Verification items for the finished model (mm, model axes). Give positions to 0.01 mm unless a question says otherwise; leave off trailing zeros. Write each loop counter-clockwise with the first axis right and the second up, starting at its lowest first coordinate (ties: lowest second). Pieces come first, ordered by that corner, then holes. Notation, with made-up numbers: M -8,3 L 44,3 A22 ccw 44,21 Z; hole C 17.25,35 d10. An arc over 180 degrees is marked long. Answer as a JSON object with one key per item and string values.
```python
from build123d import *

# Parameters (mm, degrees)
SKETCH1_R           = 2.54
BOSS_EXTRUDE1_DEPTH = 2.286
SKETCH2_W           = 25.4
SKETCH2_H           = 31.75
CUT_EXTRUDE1_DEPTH  = 2.54
FILLET1_R           = 6.35


with BuildPart() as part:
    # Sketch1 → Boss-Extrude1 (new body)
    with BuildSketch(Plane(origin=(0, 0, 0), x_dir=(1, 0, 0), z_dir=(0, 1, 0))):
        Polygon((25.4, 114.3), (0, 114.3), (0, 0), (25.4, 0), (25.4, 31.75), (69.85, 31.75), (69.85, 82.55), (25.4, 82.55), align=None)
        with Locations(Location((12.7, 95.25, 0), (0, 0, 270))):
            Circle(SKETCH1_R, mode=Mode.SUBTRACT)
        with Locations(Location((12.7, 69.85, 0), (0, 0, 270))):
            Circle(SKETCH1_R, mode=Mode.SUBTRACT)
        with Locations(Location((12.7, 44.45, 0), (0, 0, 270))):
            Circle(SKETCH1_R, mode=Mode.SUBTRACT)
        with Locations(Location((12.7, 19.05, 0), (0, 0, 270))):
            Circle(SKETCH1_R, mode=Mode.SUBTRACT)
        with Locations(Location((38.1, 69.85, 0), (0, 0, 270))):
            Circle(SKETCH1_R, mode=Mode.SUBTRACT)
        with Locations(Location((50.8, 69.85, 0), (0, 0, 270))):
            Circle(SKETCH1_R, mode=Mode.SUBTRACT)
        with Locations(Location((63.5, 69.85, 0), (0, 0, 270))):
            Circle(SKETCH1_R, mode=Mode.SUBTRACT)
        with Locations(Location((50.8, 57.15, 0), (0, 0, 270))):
            Circle(SKETCH1_R, mode=Mode.SUBTRACT)
        with Locations(Location((63.5, 57.15, 0), (0, 0, 270))):
            Circle(SKETCH1_R, mode=Mode.SUBTRACT)
        with Locations(Location((50.8, 44.45, 0), (0, 0, 270))):
            Circle(SKETCH1_R, mode=Mode.SUBTRACT)
        with Locations(Location((63.5, 44.45, 0), (0, 0, 270))):
            Circle(SKETCH1_R, mode=Mode.SUBTRACT)
        with Locations(Location((38.1, 57.15, 0), (0, 0, 270))):
            Circle(SKETCH1_R, mode=Mode.SUBTRACT)
        with Locations(Location((38.1, 44.45, 0), (0, 0, 270))):
            Circle(SKETCH1_R, mode=Mode.SUBTRACT)
    extrude(amount=BOSS_EXTRUDE1_DEPTH)

    # Sketch2 → Cut-Extrude1 (cut)
    with BuildSketch(Plane(origin=(0, 2.286, 0), x_dir=(1, 0, 0), z_dir=(0, 1, 0))):
        with Locations((12.7, 98.425)):
            Rectangle(SKETCH2_W, SKETCH2_H)
    extrude(amount=-CUT_EXTRUDE1_DEPTH, mode=Mode.SUBTRACT)

    # Fillet1
    fillet1_edges = [part.edges().sort_by_distance(p)[0] for p in [
        (69.85, 1.143, -82.55),
        (69.85, 1.143, -31.75),
        (25.4, 1.143, -31.75),
        (25.4, 1.143, 0),
        (0, 1.143, 0),
        (0, 1.143, -82.55),
    ]]
    fillet(fillet1_edges, radius=FILLET1_R)


solid = part.part
```
1) Section check B-B on z = -44.45. Record the boundary of the cut face in (x, y), and give its area (3 significant figures).
Completed:
{"outline": "M 0,0 L 10.16,0 L 10.16,2.29 L 0,2.29 Z; M 15.24,0 L 35.56,0 L 35.56,2.29 L 15.24,2.29 Z; M 40.64,0 L 48.26,0 L 48.26,2.29 L 40.64,2.29 Z; M 53.34,0 L 60.96,0 L 60.96,2.29 L 53.34,2.29 Z; M 66.04,0 L 69.85,0 L 69.85,2.29 L 66.04,2.29 Z", "area": "113 mm2"}
2) Section check C-C on y = 0.5. Count the separate pieces of the cut face and the enclosed holes in it, and give its area (3 significant figures).
Completed:
{"separate pieces": "1", "enclosed holes": "12", "area": "4,080 mm2"}
3) Thickness scan on L1, parallel to X at y = 0.6, z = -44.5; L2, parallel to X at y = 0.8, z = -57.15; L3, parallel to Z at x = 64.5, y = 2. Record the ranges inside material, lowest first.
Completed:
{"L1": "x = 0 to 10.16, 15.24 to 35.56, 40.64 to 48.26, 53.34 to 60.96, 66.04 to 69.85", "L2": "x = 0 to 35.56, 40.64 to 48.26, 53.34 to 60.96, 66.04 to 69.85", "L3": "z = -82.47 to -72.18, -67.52 to -59.48, -54.82 to -46.78, -42.12 to -31.83"}
4) Release check for a two-part mould opening along X. For faces 1 (the face through (34, 2.286, -51)), 2 (the face through (69.85, 1, -57)), 3 (the face through (38.863, 1.127, -54.727)) record: pulls with the +X half, pulls with the -X half, needs draft (parallel to the pull), parting line crosses it, or undercut.
Completed:
{"face 1": "needs draft", "face 2": "pulls with the +X half", "face 3": "undercut"}
5) Go/stop test with a flat-tipped pin: pin 1 (1.1 mm diameter, centred on x = 43, y = 0.5, fed in from +Z). Record where the tip stops, or that it passes through.
Completed:
{"pin 1": "stops at z = -31.75"}
6) Section check A-A on x = 50.8. Record the boundary of the cut face in (y, z), and give its area (3 significant figures).
Completed:
{"outline": "M 0,-82.55 L 2.29,-82.55 L 2.29,-72.39 L 0,-72.39 Z; M 0,-67.31 L 2.29,-67.31 L 2.29,-59.69 L 0,-59.69 Z; M 0,-54.61 L 2.29,-54.61 L 2.29,-46.99 L 0,-46.99 Z; M 0,-41.91 L 2.29,-41.91 L 2.29,-31.75 L 0,-31.75 Z", "area": "81.3 mm2"}
7) Section check D-D on z = -19.05. Record the boundary of the cut face in (x, y).
Completed:
{"outline": "M 0,0 L 10.16,0 L 10.16,2.29 L 0,2.29 Z; M 15.24,0 L 25.4,0 L 25.4,2.29 L 15.24,2.29 Z"}
